The listing builds one solid part. Answer for the finished solid, in the listing's coordinates (mm). Face numbers are marked on the shaded views. A direction names the side the tool comes from. Round coordinates to 2 decimals unless told otherwise and drop trailing zeros. Order: outer loops, then holes, each group sorted by start corner. A loop starts at its lowest first (then second) coordinate and runs counter-clockwise, first axis right, second up. Notation, with made-up numbers: (15.5, 8.5) - (34.5, 8.5) arc R17 cw to (34.5, 28.5) - close; hole circle Ø10 at (82.5, 51). An arc over 180 degrees is marked (long way). Write item = value, one per line.
from build123d import *

# Parameters (mm, degrees)
F1_DEPTH = 10
F3_DEPTH = 15
F4_R     = 2.5
F5_DEPTH = 12.441755


with BuildPart() as f1:
    # F0 (on Top) → F1 (new body)
    with BuildSketch(Plane.XY):
        Polygon((-13.5, -30), (13.5, -30), (13.5, 30), (-13.5, 30), (-13.5, 28), (-13.5, 24), (-11.5, 24), (-11.5, 28), (11.5, 28), (11.5, -28), (-11.5, -28), (-11.5, -24), (-13.5, -24), (-13.5, -28), align=None)
    extrude(amount=F1_DEPTH)

    # F2 (on face) → F3 (join)
    with BuildSketch(Plane(origin=(0, 30, 0), x_dir=(-1, 0, 0), z_dir=(0, 1, 0))):
        Polygon((-11.324562, 0), (-6.092738, 0), (6.730338, 10), (1.498514, 10), align=None)
    extrude(amount=F3_DEPTH)

    # F4 (on face) → F5 (cut, through all)
    with BuildSketch(Plane(origin=(2.304091, 0, 2.954554), x_dir=(0.788562, 0, -0.614955), z_dir=(-0.614955, 0, -0.788562))):
        with Locations((-2.187925, -38.680334)):
            Circle(F4_R)
    extrude(amount=-F5_DEPTH, mode=Mode.SUBTRACT)


solid = f1.part
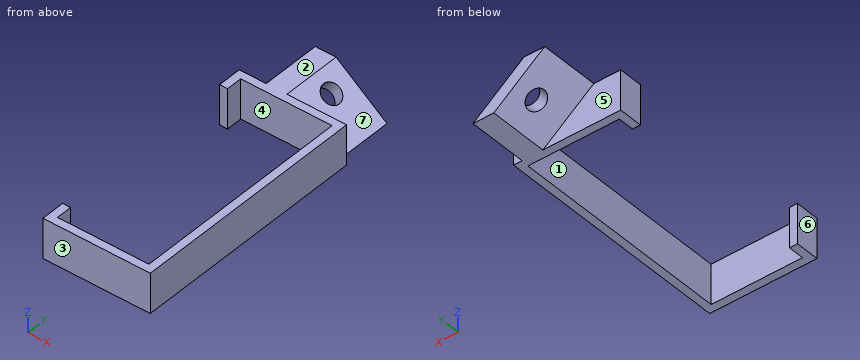
Q1. Flat-ended cylindrical pins translate along their axes: P1, Ø1.5, axis at x = -10.5, z = 6.5, coming from the +Y side; P2, Ø3, axis at y = 10, z = 4.5, coming from the -X side; P3, Ø5, axis at x = -1, z = 3.5, coming from the +Y side. Find the tip coordinate at first contact, or state that the pin passes through.
Model answer:
P1 = 30
P2 = 11.5
P3 = 45
Q2. Find the intervals of material crossed by line 1 (Y direction, x = 2, z = 9.25); line 2 (X direction, y = 27.5, z = 4.75); line 3 (Y direction, x = -12, z = 3.5), in increasing order. Write a range as from..to.
Model answer:
line_1 = -30..-28, 28..30
line_2 = -13.5..-11.5, 11.5..13.5
line_3 = -30..-24, 24..30
Q3. Determine the mould class of the marked faces 1, 2 and 3 for opening direction Y: released by +Y, released by -Y, zero draft, split by the parting line, or undercut.
Model answer:
face_1 = undercut
face_2 = zero draft
face_3 = released by -Y
Q4. For the marked faces 4, 5, 6 and 7, determine the directions among +Z, -Z, +X, -X, +Y, -Y from which every point of the face is accessible in a straight line to the end or side of a thin tool.
Model answer:
face_4 = +Z, -Z
face_5 = -Z, -X, +Y
face_6 = +Z, -Z, -X, +Y, -Y
face_7 = +Z, +X, +Y
Q5. Section B-B on z = 9.25 is taken. Determine the outline of the cut face in (x, y), then the cut area to 3 significant figures.
Model answer:
outline = (-13.5, -30) - (13.5, -30) - (13.5, 30) - (-0.54, 30) - (-0.54, 45) - (-5.77, 45) - (-5.77, 30) - (-13.5, 30) - (-13.5, 24) - (-11.5, 24) - (-11.5, 28) - (11.5, 28) - (11.5, -28) - (-11.5, -28) - (-11.5, -24) - (-13.5, -24) - close
area = 314 mm^2
Q6. Section A-A on x = -9.75 is taken. Determine the outline of the cut face in (y, z), then the cut area to 3 significant figures.
Model answer:
outline = (-30, 0) - (-28, 0) - (-28, 10) - (-30, 10) - close; (28, 0) - (30, 0) - (30, 10) - (28, 10) - close
area = 40.0 mm^2
Q7. Section C-C on x = 1.25 is taken. Count the separate pieces of the cut face and the enclosed holes in it, then the cut area to 3 significant figures.
Model answer:
separate_pieces = 3
enclosed_holes = 0
area = 82.0 mm^2
Q8. Section D-D on y = 10 is taken. Determine the outline of the cut face in (x, z).
Model answer:
outline = (11.5, 0) - (13.5, 0) - (13.5, 10) - (11.5, 10) - close
